For this review, take the finished solid that the model builds, in its own axes (mm). A direction names the side the tool comes from. Round coordinates to 2 decimals unless told otherwise and drop trailing zeros. Write each loop counter-clockwise with the first axis right and the second up, starting at its lowest first coordinate (ties: lowest second). Pieces come first, ordered by that corner, then holes. Notation, with made-up numbers: (47.5, 72.5) -> (62.5, 72.5) arc R31 cw to (62.5, 111.5) -> close; hole circle Ø9 at (-25, 2.5). An arc over 180 degrees is marked (long way). Write each question's results on one line, items separated by ' | '. Start each with the question number.
Item 1: The part is to be moulded in two halves that separate along Y. For faces 4 (the cylindrical face through (-0.3, 0.8, 96.1)), 5 (the flat face through (-3, 1.014, 116)), 6 (the cylindrical face through (-0.69, 2.02, 111.2)), say which applies: +Y half, -Y half, draft (parallel to the pull), parting line (faces both ways), or undercut.
Item 2: To check wall thickness, follow line 1 along Z through (x, y) = (0, 0.35) (3 decimals); line 2 along Z through (x, y) = (44.45, 1.35) (3 decimals); line 3 along X through (y, z) = (1.95, 63.5) (3 decimals). State the ranges of each line that lie inside material, in increasing order.
Item 3: Add section B-B (x = 38). State the section outline as (y, z) points.
Item 4: Clearance check with flat-ended pins moving along their axes: pin 1 (6.5 mm diameter, centred on x = 0, z = 115, fed in from -Y); pin 2 (1.5 mm diameter, centred on x = 26.5, y = 1, fed in from +Z). State where each tip first meets the part, or that it passes through.
Item 5: Tool access review of faces 1 (the flat face through (13.52, 1.5, 39.44)), 2 (the cylindrical face through (-0.69, 1.5, -3.1)), 3 (the cylindrical face through (-1.2, 0.5, 58.12)): name each direction out of +Z, -Z, +X, -X, +Y, -Y from which nothing blocks a thin tool from reaching the whole face with its end or side.
Item 6: Add section A-A (z = 54). State the section outline as (x, y) points, plus the area to 3 significant figures.
from build123d import *

# Parameters (mm, degrees)
F0_R     = 3.175
F0_R_2   = 1.5875
F1_DEPTH = 3.048
F2_R     = 6.2647039053
F2_R_2   = 3.175
F2_R_3   = 5.5140447668
F3_DEPTH = 1.01377
F4_R     = 1.0304590852
F5_DEPTH = 34.51469


with BuildPart() as f1:
    # F0 (on Front) → F1 (new body)
    with BuildSketch(Plane.XZ):
        with BuildLine():
            ThreePointArc((-9.4502929642, 115.490625), (-0.596483242, 104.7936951058), (9.525, 114.3))
            ThreePointArc((9.525, 114.3), (9.5063048942, 114.896483242), (9.4502929642, 115.490625))
            ThreePointArc((9.4502929642, 115.490625), (0, 123.825), (-9.4502929642, 115.490625))
        make_face()
        with Locations((0, 114.3)):
            Circle(F0_R, mode=Mode.SUBTRACT)
        with BuildLine():
            ThreePointArc((52.3875, 0), (50.1616327839, 5.5119104847), (44.7324052746, 7.9324746146))
            ThreePointArc((44.7324052746, 7.9324746146), (36.5125, 0), (44.7324052746, -7.9324746146))
            ThreePointArc((44.7324052746, -7.9324746146), (50.1616327839, -5.5119104847), (52.3875, 0))
        make_face()
        with Locations((44.45, 0)):
            Circle(F0_R, mode=Mode.SUBTRACT)
        with BuildLine():
            ThreePointArc((9.4502929642, 115.490625), (9.5063048942, 114.896483242), (9.525, 114.3))
            ThreePointArc((9.525, 114.3), (-0.596483242, 104.7936951058), (-9.4502929642, 115.490625))
            Line((-9.4502929642, 115.490625), (-15.7504882737, 65.484375))
            ThreePointArc((-15.7504882737, 65.484375), (0, 79.375), (15.7504882737, 65.484375))
            Line((15.7504882737, 65.484375), (9.4502929642, 115.490625))
        make_face()
        with Locations((-2.209718572, 100.0252)):
            Circle(F0_R_2, mode=Mode.SUBTRACT)
        with BuildLine():
            ThreePointArc((15.875, 63.5), (15.8438414904, 64.4941387366), (15.7504882737, 65.484375))
            ThreePointArc((15.7504882737, 65.484375), (0, 79.375), (-15.7504882737, 65.484375))
            ThreePointArc((-15.7504882737, 65.484375), (-15.8721860132, 63.2011084429), (-15.6646119555, 60.9240424533))
            ThreePointArc((-15.6646119555, 60.9240424533), (0.4924504072, 47.6326398668), (15.7942028036, 61.9003804205))
            ThreePointArc((15.7942028036, 61.9003804205), (15.8547878338, 62.6991705884), (15.875, 63.5))
        make_face()
        with Locations((0, 63.5)):
            Circle(F0_R, mode=Mode.SUBTRACT)
        with BuildLine():
            ThreePointArc((15.7942028036, 61.9003804205), (0.4924504072, 47.6326398668), (-15.6646119555, 60.9240424533))
            Line((-15.6646119555, 60.9240424533), (-9.525, 0))
            ThreePointArc((-9.525, 0), (0, 9.525), (9.525, 0))
            ThreePointArc((9.525, 0), (6.9705567315, -6.4912990883), (0.6773435479, -9.500885786))
            Line((0.6773435479, -9.500885786), (44.7324052746, -7.9324746146))
            ThreePointArc((44.7324052746, -7.9324746146), (36.5125, 0), (44.7324052746, 7.9324746146))
            Line((44.7324052746, 7.9324746146), (18.9341027877, 8.850924033))
            ThreePointArc((18.9341027877, 8.850924033), (13.2249738114, 11.5709798305), (11.3072231466, 17.5971800924))
            Line((11.3072231466, 17.5971800924), (15.7942028036, 61.9003804205))
        make_face()
        with BuildLine():
            ThreePointArc((9.525, 0), (0, 9.525), (-9.525, 0))
            ThreePointArc((-9.525, 0), (-6.7351920908, -6.7351920908), (0, -9.525))
            Line((0, -9.525), (0.6773435479, -9.500885786))
            ThreePointArc((0.6773435479, -9.500885786), (6.9705567315, -6.4912990883), (9.525, 0))
        make_face()
        Circle(F0_R, mode=Mode.SUBTRACT)
        with BuildLine():
            Line((0.6773435479, -9.500885786), (0, -9.525))
            ThreePointArc((0, -9.525), (0.3388863295, -9.5189695375), (0.6773435479, -9.500885786))
        make_face()
    extrude(amount=-F1_DEPTH)

    # F2 (on face) → F3 (cut)
    with BuildSketch(Plane.XZ):
        with Locations((0, 114.3)):
            Circle(F2_R)
        with Locations((0, 114.3)):
            Circle(F2_R_2, mode=Mode.SUBTRACT)
        with Locations((0, 63.5)):
            Circle(F2_R_3)
        with Locations((0, 63.5)):
            Circle(F2_R_2, mode=Mode.SUBTRACT)
    extrude(amount=-F3_DEPTH, mode=Mode.SUBTRACT)

    # F4 (on face) → F5 (cut)
    with BuildSketch(Plane(origin=(23.6257324105, 0, 2.9765625), x_dir=(0, 1, 0), z_dir=(0.9921567416, 0, 0.125))):
        with Locations((1.524, 66.0321041942)):
            Circle(F4_R)
        with Locations((1.524, 74.8308971524)):
            Circle(F4_R)
        with Locations((1.524, 82.4269801378)):
            Circle(F4_R)
        with Locations((1.524, 94.6481488792)):
            Circle(F4_R)
        with Locations((1.524, 106.101423502)):
            Circle(F4_R)
    extrude(amount=-F5_DEPTH, mode=Mode.SUBTRACT)


solid = f1.part
Responses:
1) face 4: undercut | face 5: -Y half | face 6: draft
2) line 1: z = -9.525 to -3.175, 3.175 to 57.986, 69.014 to 108.035, 120.565 to 123.825 | line 2: z = -7.943 to -3.175, 3.175 to 7.943 | line 3: x = -15.875 to -3.175, 3.175 to 15.875
3) outline: (0, -8.17) -> (3.05, -8.17) -> (3.05, 8.17) -> (0, 8.17) -> close
4) pin 1: stops at y = 1.01 | pin 2: stops at z = 8.61
5) face 1: +X, +Y, -Y | face 2: +Y, -Y | face 3: -Y
6) outline: (-14.97, 0) -> (14.99, 0) -> (14.99, 3.05) -> (-14.97, 3.05) -> close | area: 91.3 mm^2
